```python
from build123d import *

# Parameters (mm, degrees)
SALIENTE_EXTRUIR1_DEPTH = 3
CROQUIS2_R              = 2.25
CROQUIS2_R_2            = 3.25
CORTAR_EXTRUIR1_DEPTH   = 3


with BuildPart() as part:
    # Croquis1 → Saliente-Extruir1 (new body)
    with BuildSketch(Plane.XY):
        with BuildLine():
            Line((-23.25, 9.768613172), (23.25, 9.768613172))
            ThreePointArc((23.25, 9.768613172), (33.25, -0.231386828), (23.25, -10.231386828))
            Line((23.25, -10.231386828), (-23.25, -10.231386828))
            ThreePointArc((-23.25, -10.231386828), (-33.25, -0.231386828), (-23.25, 9.768613172))
        make_face()
    extrude(amount=SALIENTE_EXTRUIR1_DEPTH)

    # Croquis2 → Cortar-Extruir1 (cut)
    with BuildSketch(Plane(origin=(0, 0, 0), x_dir=(-1, 0, 0), z_dir=(0, 0, -1))):
        with Locations((14, 0)):
            Circle(CROQUIS2_R)
        with Locations((27, 0)):
            Circle(CROQUIS2_R)
        with Locations((-23.25, 0)):
            Circle(CROQUIS2_R_2)
    extrude(amount=-CORTAR_EXTRUIR1_DEPTH, mode=Mode.SUBTRACT)


solid = part.part
```
Model file for the job. Use its own axes, mm. Coordinates: 2 decimals unless noted, no trailing zeros. Loops run counter-clockwise (first coordinate to the right, second up) from the corner with the lowest first, then second, coordinate; pieces in that order, holes last. Notation, with made-up numbers: (42, -4) - (98, -4) arc R34 ccw to (98, 30) - close; hole circle Ø8 at (-38, 81.25). An arc over 180 degrees is marked (long way). Answer as a JSON object with one key per item and string values. Group by question number.
(1) Probe line 1 along X through (y, z) = (-0.5, 2.6); line 2 along X through (y, z) = (-2.75, 0.95); line 3 along Y through (x, z) = (-28, 2.3). List the from-to ranges inside material, lowest first.
(2) Cut at A-A (z = 1.25). Give the cut face in (x, y), then the cut area to 3 significant figures.
(3) Cut at C-C (y = 0.75). Give the cut face in (x, z).
(4) Two-plate mould, pull along X, no slides. Class faces 1 (the face through (-33.248, -0.451, 1.479)), 2 (the face through (-16.146, 0.676, 1.479)), 3 (the face through (0, -10.231, 1)): released by +X, released by -X, zero draft, split by the parting line, or undercut.
(5) Cut at D-D (x = -28). Give the cut face in (y, z), then the cut area to 3 significant figures.
(6) Flat gauge pin, fed straight in: pin 1 (5 mm diameter, centred on x = 23.25, y = 0, fed in from -Z). Where does the tip first touch, or does it go through?
(7) Cut at B-B (x = -14). Give the cut face in (y, z).
Geometry says:
{
 "1": {"line 1": "x = -33.25 to -29.19, -24.81 to -16.19, -11.81 to 20.04, 26.46 to 33.25", "line 2": "x = -32.93 to 21.52, 24.98 to 32.93", "line 3": "y = -9.03 to -2.02, 2.02 to 8.57"},
 "2": {"outline": "(-23.25, -10.23) - (23.25, -10.23) arc R10 ccw to (23.25, 9.77) - (-23.25, 9.77) arc R10 ccw to start; hole circle Ø4.5 at (-27, 0); hole circle Ø4.5 at (-14, 0); hole circle Ø6.5 at (23.25, 0)", "area": "1,180 mm^2"},
 "3": {"outline": "(-33.2, 0) - (-29.12, 0) - (-29.12, 3) - (-33.2, 3) - close; (-24.88, 0) - (-16.12, 0) - (-16.12, 3) - (-24.88, 3) - close; (-11.88, 0) - (20.09, 0) - (20.09, 3) - (-11.88, 3) - close; (26.41, 0) - (33.2, 0) - (33.2, 3) - (26.41, 3) - close"},
 "4": {"face 1": "released by -X", "face 2": "undercut", "face 3": "zero draft"},
 "5": {"outline": "(-9.03, 0) - (-2.02, 0) - (-2.02, 3) - (-9.03, 3) - close; (2.02, 0) - (8.57, 0) - (8.57, 3) - (2.02, 3) - close", "area": "40.7 mm^2"},
 "6": {"pin 1": "passes through"},
 "7": {"outline": "(-10.23, 0) - (-2.25, 0) - (-2.25, 3) - (-10.23, 3) - close; (2.25, 0) - (9.77, 0) - (9.77, 3) - (2.25, 3) - close"}
}
